Part model, mm, in its own coordinate system. A direction names the side the tool comes from. Round coordinates to 2 decimals unless told otherwise and drop trailing zeros. Write each loop counter-clockwise with the first axis right and the second up, starting at its lowest first coordinate (ties: lowest second). Pieces come first, ordered by that corner, then holes.
Autodesk Inventor part; units mm, degrees
ref_plane "YZ Plane" through (0, 0, 0) normal (1, 0, 0) x (0, 1, 0)
ref_plane "XZ Plane" through (0, 0, 0) normal (0, 1, 0) x (-1, 0, 0)
ref_plane "XY Plane" through (0, 0, 0) normal (0, 0, 1) x (1, 0, 0)
sketch "Sketch1" plane through (0, 0, 0) normal (0, 1, 0) x (-1, 0, 0)
  circle A0 centre (130.4354, 61.1321) radius 1.4224
  point P0 (0, 0)
  dimension "d0" = 2.8448
extrude "Extrusion1" add sketch "Sketch1" along normal blind 6.35
sketch "Sketch2" plane through (-130.4354, 0, 61.1321) normal (0, -1, 0) x (1, 0, 0)
  circle A0 centre (0, 0) radius 1.4224 construction
  line L0 (3.1527, 5.5122) -> (6.35, 0.0258)
  line L1 (6.35, 0.0258) -> (3.1973, -5.4864)
  line L2 (3.1973, -5.4864) -> (-3.1527, -5.5122)
  line L3 (-3.1527, -5.5122) -> (-6.35, -0.0258)
  line L4 (-6.35, -0.0258) -> (-3.1973, 5.4864)
  line L5 (-3.1973, 5.4864) -> (3.1527, 5.5122)
  point P0 (130.4354, -61.1321)
  dimension "d3" = 6.35
extrude "Extrusion2" add sketch "Sketch2" along normal blind 25.4
sketch "Sketch3" plane through (-130.4354, -25.4, 61.1321) normal (0, -1, 0) x (1, 0, 0)
  circle A0 centre (0, 0) radius 1.4224
  point P0 (130.4354, -61.1321)
extrude "Extrusion3" add sketch "Sketch3" along normal blind 6.35
Q1. Saw through at A-A, the plane y = -12. Write the cut outline in (x, z).
Q2. Tool access for faces 1 (the flat face through (-130, -31.75, 61)), 2 (the flat face through (-129, 0, 60)), 3 (the flat face through (-129, -25.4, 60)): list every direction of +Z, -Z, +X, -X, +Y, -Y with a clear straight run to the whole face (end or side of a thin tool).
Q3. Saw through at C-C, the plane z = 62. Write the cut outline in (x, y).
Q4. Saw through at D-D, the plane z = 64.75. Write the cut outline in (x, y).
Q5. Saw through at B-B, the plane x = -130.5. Write the cut outline in (y, z), and give its area (3 significant figures).
Q6. Wall check: line 1 (Y direction, x = -131.75, z = 66.25); line 2 (Z direction, x = -129.5, y = -11); line 3 (X direction, y = -3.5, z = 63). Give the ranges that are in metal, low to high.
Q7. Drop flat-ended pins along their axis: P1, Ø5, axis at y = -19.5, z = 63.5, coming from the -X side; P2, Ø2, axis at x = -133, z = 61, coming from the +Y side; P3, Ø6, axis at y = -13, z = 65, coming from the -X side; P4, Ø3, axis at y = -15.5, z = 60.5, coming from the +X side. Give the stop position or say it passes through.
Computed:
1. outline: (-136.79, 61.11) - (-133.59, 55.62) - (-127.24, 55.65) - (-124.09, 61.16) - (-127.28, 66.64) - (-133.63, 66.62) - close
2. face 1: +Z, -Z, +X, -X, -Y
2. face 2: +Y
2. face 3: -Y
3. outline: (-136.27, -25.4) - (-131.56, -25.4) - (-131.56, -31.75) - (-129.31, -31.75) - (-129.31, -25.4) - (-124.58, -25.4) - (-124.58, 0) - (-129.31, 0) - (-129.31, 6.35) - (-131.56, 6.35) - (-131.56, 0) - (-136.27, 0) - close
4. outline: (-134.7, -25.4) - (-126.18, -25.4) - (-126.18, 0) - (-134.7, 0) - close
5. outline: (-31.75, 59.71) - (-25.4, 59.71) - (-25.4, 55.63) - (0, 55.63) - (0, 59.71) - (6.35, 59.71) - (6.35, 62.55) - (0, 62.55) - (0, 66.63) - (-25.4, 66.63) - (-25.4, 62.55) - (-31.75, 62.55) - close
5. area: 315 mm2
6. line 1: y = -25.4 to 0
6. line 2: z = 55.64 to 66.64
6. line 3: x = -135.7 to -125.16
7. P1: stops at x = -136.79
7. P2: stops at y = 0
7. P3: stops at x = -136.27
7. P4: stops at x = -124.09
